Autodesk Inventor part; units mm, degrees
ref_plane "YZ Plane" through (0, 0, 0) normal (1, 0, 0) x (0, 1, 0)
ref_plane "XZ Plane" through (0, 0, 0) normal (0, 1, 0) x (-1, 0, 0)
ref_plane "XY Plane" through (0, 0, 0) normal (0, 0, 1) x (1, 0, 0)
sketch "Skizze1" plane through (0, 0, 0) normal (0, 0, 1) x (1, 0, 0)
  line L0 (-10.5, 0) -> (10.5, 0)
  line L1 (0, -10.5) -> (0, 10.5)
  circle A0 centre (0, 0) radius 7.5
  circle A1 centre (0, 0) radius 3
  dimension "d0" = 15
  dimension "d1" = 6
extrude "Extrusion1" add sketch "Skizze1" along normal mid plane 5 contours A1 L1 A0 L0 | L0 A0 L1 A1 | A1 L0 A0 L1 | L1 A0 L0 A1
sketch "Skizze2" plane through (0, 0, 2.5) normal (0, 0, 1) x (1, 0, 0)
  circle A0 centre (0, 0) radius 3
  circle A1 centre (0, 0) radius 7.5
  circle A2 centre (0, 0) radius 4
  circle A3 centre (0, 0) radius 6.5
  dimension "d4" = 8
  dimension "d5" = 13
extrude "Extrusion2" cut sketch "Skizze2" against normal blind 0.2 contours A3
mirror "Spiegeln1" about plane through (0, 0, 0) normal (0, 0, 1) of "Extrusion2"
chamfer "Fase1" distance 0.05 angle 45 1 edges at (-6.5, 0, 2.5)
chamfer "Fase2" distance 0.05 angle 45 1 edges at (-4, 0, 2.5)
chamfer "Fase3" distance 0.05 angle 45 1 edges at (-3, 0, 2.5)
chamfer "Fase4" distance 0.05 angle 45 1 edges at (-7.5, 0, 2.5)
chamfer "Fase5" distance 0.05 angle 45 1 edges at (-7.5, 0, -2.5)
chamfer "Fase6" distance 0.05 angle 45 1 edges at (-6.5, 0, -2.5)
chamfer "Fase7" distance 0.05 angle 45 1 edges at (-4, 0, -2.5)
chamfer "Fase8" distance 0.05 angle 45 1 edges at (-3, 0, -2.5)
properties part number "Kugellager_6x15x5_696ZZ" material "Stahl, Kohlenstoff"
The model under review builds one solid part; all positions refer to its coordinate system, in mm. A direction names the side the tool comes from. Give positions to 0.01 mm unless a question says otherwise; leave off trailing zeros. Write each loop counter-clockwise with the first axis right and the second up, starting at its lowest first coordinate (ties: lowest second). Pieces come first, ordered by that corner, then holes. Notation, with made-up numbers: M 84.25,55.5 L 118.25,55.5 A4 ccw 118.25,60.5 Z; hole C 11,19 d4. An arc over 180 degrees is marked long. Write item = value, one per line. Start each with the question number.
Q1. Machinability: for faces 1 (the face through (-3, 0, 0)), 2 (the face through (-3, 3, -2.3)), which of the approach directions +Z, -Z, +X, -X, +Y, -Y give a long, thin tool a straight path to every point of the face, cutting with its end or side? Answer none if there is none.
Q2. Clearance check with flat-ended pins moving along their axes: pin 1 (2 mm diameter, centred on x = 2.5, z = 1, fed in from +Y); pin 2 (1.5 mm diameter, centred on x = -3.5, z = -0.5, fed in from +Y); pin 3 (2 mm diameter, centred on y = -2.5, z = -1, fed in from -X). State where each tip first meets the part, or that it passes through.
Q3. Mouldability with a two-part tool opening along X and no side actions: class faces 3 (the face through (3, 3, 2.3)), 4 (the face through (2, -3, 2.5)), 5 (the face through (-7.493, 0.33, 0.034)) as released by +X, released by -X, zero draft, split by the parting line, or undercut.
Q4. We need section A-A (z = 1.1). State the section outline as (x, y) points, plus the area to 3 significant figures.
Q5. For line 1 (Y direction, x = 0, z = -2.4); line 2 (Y direction, x = 0, z = 0.9), list the stretches that pass through material, from the lowest coordinate up.
Result set:
q1.face_1 = +Z, -Z
q1.face_2 = -Z
q2.pin_1 = 7.35
q2.pin_2 = 6.98
q2.pin_3 = -7.35
q3.face_3 = undercut
q3.face_4 = zero draft
q3.face_5 = split by the parting line
q4.outline = C 0,0 d15; hole C 0,0 d6
q4.area = 148 mm2
q5.line_1 = -7.5 to -6.5, -4 to -3, 3 to 4, 6.5 to 7.5
q5.line_2 = -7.5 to -3, 3 to 7.5
